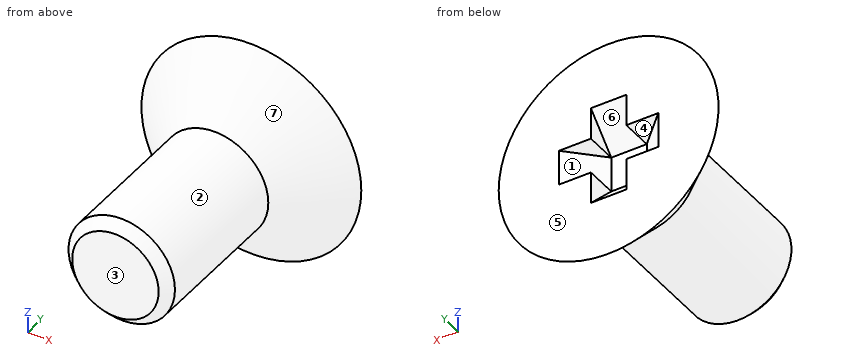
```python
from build123d import *

# Parameters (mm, degrees)
CHAMFER_1_SIZE           = 0.2805
CUT_EXTRUDE_1_DEPTH      = 0.5
PATTERN_CIRCULAR_1_COUNT = 4
SKETCH_3_W               = 1
SKETCH_3_H               = 1
EXTRUDE_1_DEPTH          = 2


with BuildPart() as part:
    # Sketch 1 → Revolve 1 (revolve)
    with BuildSketch(Plane.XY):
        Polygon((0, 0), (3.1, 0), (1.5, -1.6), (1.5, -6), (0, -6), align=None)
    revolve(axis=Axis((0, 0, 0), (0, -1, 0)))

    # Chamfer 1
    chamfer_1_edges = [part.edges().sort_by_distance(p)[0] for p in [
        (-1.5, -6, 0),
    ]]
    chamfer(chamfer_1_edges, length=CHAMFER_1_SIZE)

    # Sketch 2 → Cut-Extrude 1 (cut, symmetric)
    with BuildSketch(Plane.XY):
        Polygon((0, 0), (0, -1.4), (-1.4, 0), align=None)
    cut_extrude_1 = extrude(amount=CUT_EXTRUDE_1_DEPTH, both=True, mode=Mode.SUBTRACT)

    # Pattern Circular 1: Cut-Extrude 1 ×4 about axis
    pattern_circular_1_axis = Axis((0, 0, 0), (0, 1, 0))
    for i in range(1, PATTERN_CIRCULAR_1_COUNT):
        add(cut_extrude_1.rotate(pattern_circular_1_axis, i * 360 / PATTERN_CIRCULAR_1_COUNT), mode=Mode.SUBTRACT)

    # Sketch 3 → Extrude 1 (add)
    with BuildSketch(Plane(origin=(0, -0.9, 0), x_dir=(1, 0, 0), z_dir=(0, 1, 0))):
        Rectangle(SKETCH_3_W, SKETCH_3_H)
    extrude(amount=-EXTRUDE_1_DEPTH)


solid = part.part
```
Design review of the part built by this model. Coordinates are the model's own, in mm. Face numbers are marked on the shaded views. A direction names the side the tool comes from. Coordinates: 2 decimals unless noted, no trailing zeros. Loops run counter-clockwise (first coordinate to the right, second up) from the corner with the lowest first, then second, coordinate; pieces in that order, holes last. Notation, with made-up numbers: (74.5, -15) - (122.5, -15) arc R10 cw to (122.5, -6) - close; hole circle Ø5 at (17, -36.75). An arc over 180 degrees is marked (long way). Use CSV: the item, a comma, the result in double quotes. Start each with the question number.
1) Wall thickness on L1, parallel to Y at x = 2.25, z = 1.5; L2, parallel to X at y = -5.3, z = 1.25; L3, parallel to Z at x = 0, y = -3.2: over which ranges is each line inside the solid? List them lowest first. Write a range as from..to.
2) Consider section B-B on x = 0. Write out the cut boundary in (y, z), then the cut area to 3 significant figures.
3) Consider section D-D on y = -4.05. Write out the cut boundary in (x, z).
4) Consider section A-A on z = 0. Write out the cut boundary in (x, y).
5) Tool access review of the marked faces 1, 2 and 3: name each direction out of +Z, -Z, +X, -X, +Y, -Y from which nothing blocks a thin tool from reaching the whole face with its end or side.
6) For pin 1 Ø1 at (x, z) = (1, 1.5) entering from +Y; pin 2 Ø0.5 at (x, z) = (0, 0) entering from +Y; pin 3 Ø1 at (x, y) = (1, -0.5) entering from -Z; pin 4 Ø0.7 at (x, y) = (1, -0.5) entering from +Z, all flat-tipped, find the tip position at first contact; note any pin that passes through.
7) Consider section C-C on y = -1.2. Write out the cut boundary in (x, z).
8) The part is to be moulded in two halves that separate along X. For the marked faces 4, 5, 6 and 7, say which applies: +X half, -X half, draft (parallel to the pull), parting line (faces both ways), or undercut.
Geometry says:
1,L1,"-0.4..0"
1,L2,"-0.83..0.83"
1,L3,"-1.5..1.5"
2,outline,"(-6, -1.22) - (-5.72, -1.5) - (-1.6, -1.5) - (0, -3.1) - (0, -1.4) - (-0.9, -0.5) - (-0.9, 0.5) - (0, 1.4) - (0, 3.1) - (-1.6, 1.5) - (-5.72, 1.5) - (-6, 1.22) - close"
2,area,"18.8 mm^2"
3,outline,"circle Ø3 at (0, 0)"
4,outline,"(-3.1, 0) - (-1.5, -1.6) - (-1.5, -5.72) - (-1.22, -6) - (1.22, -6) - (1.5, -5.72) - (1.5, -1.6) - (3.1, 0) - (1.4, 0) - (0.5, -0.9) - (-0.5, -0.9) - (-1.4, 0) - close"
5,face 1,"+Y"
5,face 2,"-Y"
5,face 3,"+Z, -Z, +X, -X, -Y"
6,pin 1,"y = 0"
6,pin 2,"y = -0.9"
6,pin 3,"z = -2.96"
6,pin 4,"z = 2.79"
7,outline,"circle Ø3.8 at (0, 0)"
8,face 4,"undercut"
8,face 5,"draft"
8,face 6,"undercut"
8,face 7,"parting line"
